The drawing under review shows one solid part. Ordinate dimensions are in mm from its lowest x, y, z. A direction names the side the tool comes from. Coordinates: 2 decimals unless noted, no trailing zeros. Loops run counter-clockwise (first coordinate to the right, second up) from the corner with the lowest first, then second, coordinate; pieces in that order, holes last.
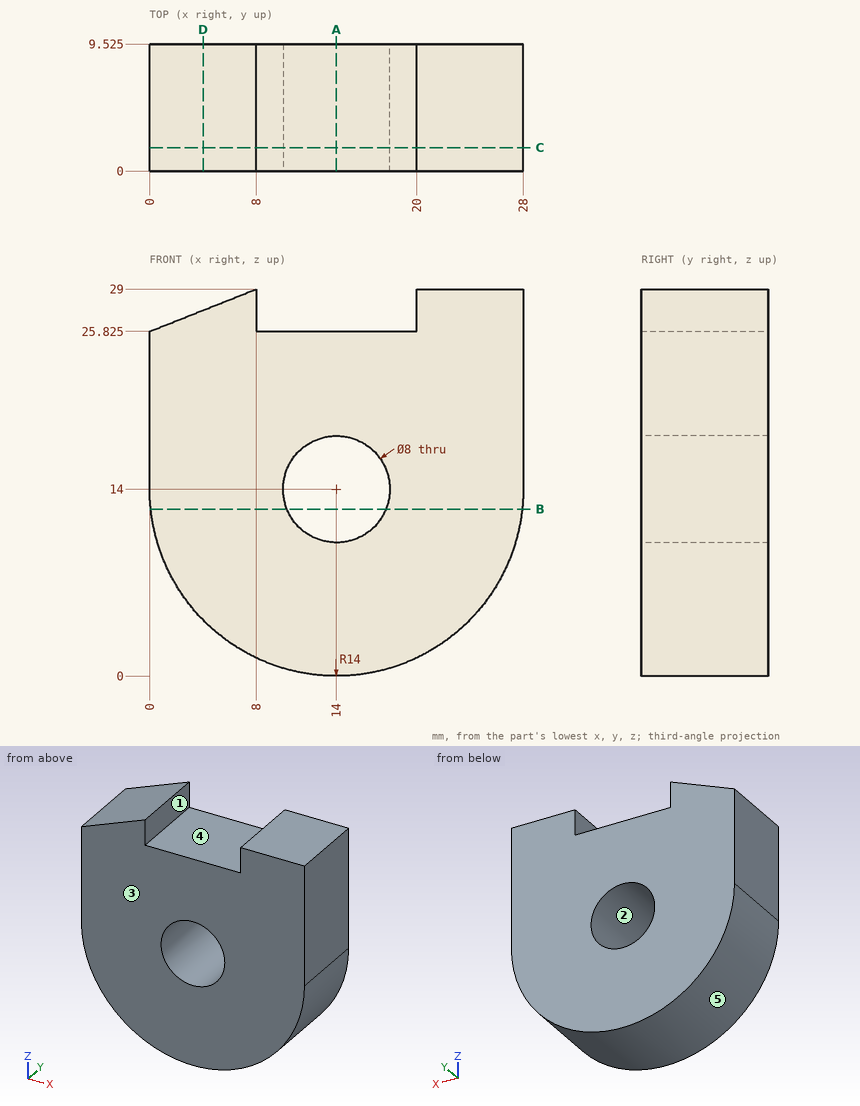
Q1. The part is to be moulded in two halves that separate along X. For the marked faces 3, 4 and 5, say which applies: pulls with the +X half, pulls with the -X half, needs draft (parallel to the pull), parting line crosses it, or undercut.
Q2. Take a section at A-A, the plane x = 14. Write out the cut boundary in (y, z) (3 decimals), then the cut area to 3 significant figures.
Q3. Clearance check with flat-ended pins moving along their axes: pin 1 Ø4 at (x, y) = (8, 4) entering from +Z; pin 2 Ø1 at (x, y) = (5, 6.5) entering from +Z; pin 3 Ø5 at (x, y) = (5, 6) entering from +Z. State where each tip first meets the part, or that it passes through.
Q4. For line 1 (X direction, y = 3.75, z = 14); line 2 (Z direction, x = 14, y = 7.25) (3 decimals); line 3 (X direction, y = 6.25, z = 11.75), list the stretches that pass through material, from the lowest coordinate up.
Q5. Take a section at B-B, the plane z = 12.5. Write out the cut boundary in (x, y) (3 decimals).
Q6. Machinability: for the marked faces 1 and 2, which of the approach directions +Z, -Z, +X, -X, +Y, -Y give a long, thin tool a straight path to every point of the face, cutting with its end or side? Answer none if there is none.
Q7. Take a section at D-D, the plane x = 4. Write out the cut boundary in (y, z) (1 decimal), then the cut area to 3 significant figures.
Q8. Take a section at C-C, the plane y = 1.75. Write out the cut boundary in (x, z) (3 decimals), then the cut area to 3 significant figures.
Entries:
1. face 3: needs draft
1. face 4: undercut
1. face 5: parting line crosses it
2. outline: (0, 0) - (9.525, 0) - (9.525, 10) - (0, 10) - close; (0, 18) - (9.525, 18) - (9.525, 25.825) - (0, 25.825) - close
2. area: 170 mm2
3. pin 1: stops at z = 29
3. pin 2: stops at z = 28.01
3. pin 3: stops at z = 28.8
4. line 1: x = 0 to 10, 18 to 28
4. line 2: z = 0 to 10, 18 to 25.825
4. line 3: x = 0.18 to 10.69, 17.31 to 27.82
5. outline: (0.081, 0) - (10.292, 0) - (10.292, 9.525) - (0.081, 9.525) - close; (17.708, 0) - (27.919, 0) - (27.919, 9.525) - (17.708, 9.525) - close
6. face 1: +Z, +Y, -Y
6. face 2: +Y, -Y
7. outline: (0, 4.2) - (9.5, 4.2) - (9.5, 27.4) - (0, 27.4) - close
7. area: 221 mm2
8. outline: (0, 14) arc R14 ccw to (28, 14) - (28, 29) - (20, 29) - (20, 25.825) - (8, 25.825) - (8, 29) - (0, 25.825) - close; hole circle Ø8 at (14, 14)
8. area: 627 mm2
